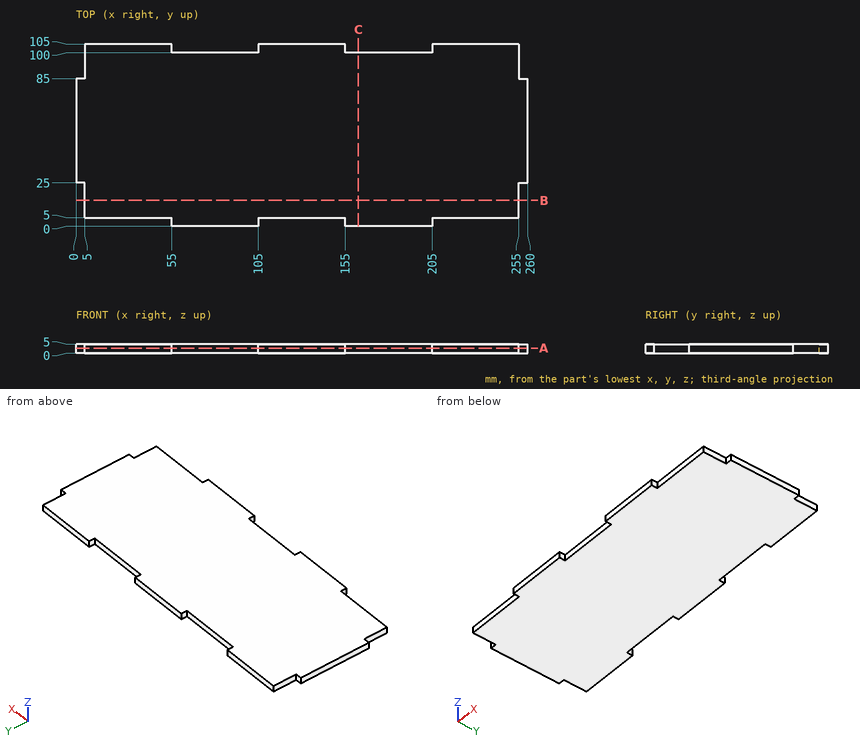
Input: dimensioned drawing with shaded views. Units: mm. Origin: part minimum x, y, z. Coordinates: 2 decimals unless noted, no trailing zeros. Order: outer loops, then holes, each group sorted by start corner. A loop starts at its lowest first (then second) coordinate and runs counter-clockwise, first axis right, second up. Notation, with made-up numbers: (23, -24) -> (77, -24) arc R13 cw to (77, -14) -> close; hole circle Ø11 at (15, 69). An arc over 180 degrees is marked (long way). Use CSV: the item, a comma, the result in double quotes.
1) Section A-A on z = 2.85. Output: boundary loops of the cut face in (x, y).
Findings:
outline,"(0, 25) -> (5, 25) -> (5, 5) -> (55, 5) -> (55, 0) -> (105, 0) -> (105, 5) -> (155, 5) -> (155, 0) -> (205, 0) -> (205, 5) -> (255, 5) -> (255, 25) -> (260, 25) -> (260, 85) -> (255, 85) -> (255, 105) -> (205, 105) -> (205, 100) -> (155, 100) -> (155, 105) -> (105, 105) -> (105, 100) -> (55, 100) -> (55, 105) -> (5, 105) -> (5, 85) -> (0, 85) -> close"
2) Line query: line 1 (Y direction, x = 40, z = 1.3); line 2 (X direction, y = 14, z = 1.1); line 3 (Y direction, x = 196.5, z = 2.65). Output: solid intervals per line, ascending.
Findings:
line 1,"y = 5 to 105"
line 2,"x = 5 to 255"
line 3,"y = 0 to 100"
3) Pin query (flat end, axial travel): pin 1 Ø2.5 at (x, z) = (29.5, 2) entering from -Y; pin 2 Ø1.5 at (x, y) = (162.5, 43) entering from -Z; pin 3 Ø1.5 at (x, z) = (2, 3.5) entering from +Y; pin 4 Ø1.5 at (y, z) = (3.5, 3) entering from -X. Return the tip coordinate at first contact, or that it passes through.
Findings:
pin 1,"stops at y = 5"
pin 2,"stops at z = 0"
pin 3,"stops at y = 85"
pin 4,"stops at x = 55"
4) Section B-B on y = 15. Output: boundary loops of the cut face in (x, z).
Findings:
outline,"(5, 0) -> (255, 0) -> (255, 5) -> (5, 5) -> close"
5) Section C-C on x = 162.5. Output: boundary loops of the cut face in (y, z).
Findings:
outline,"(0, 0) -> (100, 0) -> (100, 5) -> (0, 5) -> close"
